Geometry: final body of the model. Coordinates: model frame, mm. Coordinates: 2 decimals unless noted, no trailing zeros. Loops run counter-clockwise (first coordinate to the right, second up) from the corner with the lowest first, then second, coordinate; pieces in that order, holes last. Notation, with made-up numbers: M -13.5,-37.75 L 44.5,-37.75 A19 ccw 44.5,-13.75 Z; hole C 77,2 d6. An arc over 180 degrees is marked long. Write item = value, one per line. Start each with the question number.
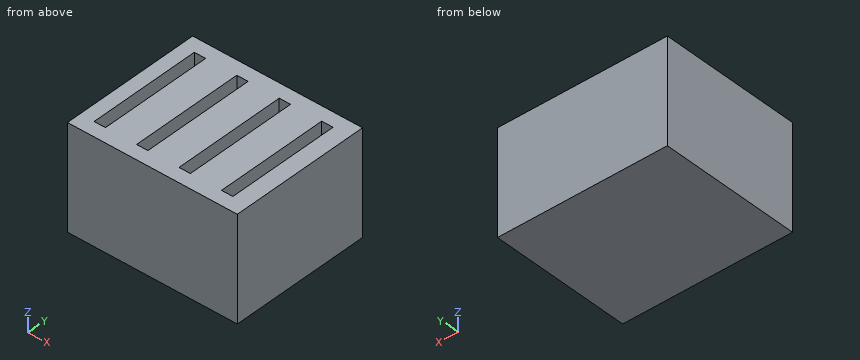
```python
from build123d import *

# Parameters (mm, degrees)
BOX_W        = 2.4
BOX_H        = 24
BOX_DEPTH    = 22
BOX001_W     = 2.4
BOX001_H     = 24
BOX001_DEPTH = 22
BOX002_W     = 2.4
BOX002_H     = 24
BOX002_DEPTH = 22
BOX003_W     = 2.4
BOX003_H     = 24
BOX003_DEPTH = 22
BOX004_W     = 36
BOX004_H     = 30
BOX004_DEPTH = 22


with BuildPart() as box:
    # Box → Box (new body)
    with BuildSketch(Plane.XY):
        with Locations((1.2, 12)):
            Rectangle(BOX_W, BOX_H)
    extrude(amount=BOX_DEPTH)


with BuildPart() as box001:
    # Box001 → Box001 (new body)
    with BuildSketch(Plane(origin=(9, 0, 0), x_dir=(1, 0, 0), z_dir=(0, 0, 1))):
        with Locations((1.2, 12)):
            Rectangle(BOX001_W, BOX001_H)
    extrude(amount=BOX001_DEPTH)


with BuildPart() as box002:
    # Box002 → Box002 (new body)
    with BuildSketch(Plane(origin=(18, 0, 0), x_dir=(1, 0, 0), z_dir=(0, 0, 1))):
        with Locations((1.2, 12)):
            Rectangle(BOX002_W, BOX002_H)
    extrude(amount=BOX002_DEPTH)


with BuildPart() as ranuras:
    # Box003 → Box003 (new body)
    with BuildSketch(Plane(origin=(27, 0, 0), x_dir=(1, 0, 0), z_dir=(0, 0, 1))):
        with Locations((1.2, 12)):
            Rectangle(BOX003_W, BOX003_H)
    extrude(amount=BOX003_DEPTH)

    # Fusion: union Box, Box001, Box002
    add(box.part)
    add(box001.part)
    add(box002.part)


with BuildPart() as ranuras_1:
    # Fusion placement: moved
    add(ranuras.part.moved(Location((0, 0, 3))))


with BuildPart() as cut:
    # Box004 → Box004 (new body)
    with BuildSketch(Plane(origin=(-3, -3, 0), x_dir=(1, 0, 0), z_dir=(0, 0, 1))):
        with Locations((18, 15)):
            Rectangle(BOX004_W, BOX004_H)
    extrude(amount=BOX004_DEPTH)

    # Cut: cut Ranuras
    add(ranuras_1.part, mode=Mode.SUBTRACT)


solid = cut.part
```
Item 1: First-contact query: pin 1 (1.9 mm diameter, centred on x = 28.5, y = 13, fed in from +Z); pin 2 (0.7 mm diameter, centred on x = 10, y = 13, fed in from +Z). Flat tips, straight axial feed; report the tip coordinate or a pass-through.
Item 2: Section query A-A (z = 13.25). Return the cut outline in (x, y), plus the area to 3 significant figures.
Item 3: Line query: line 1 (X direction, y = 8, z = 16.75); line 2 (Y direction, x = 10, z = 15.75). Output: solid intervals per line, ascending. Write a range as from..to.
Item 4: Section query B-B (y = 12.75). Return the cut outline in (x, z).
Item 5: Section query C-C (x = 28.5). Return the cut outline in (y, z), plus the area to 3 significant figures.
Verdict:
q1.pin_1 = 22
q1.pin_2 = 3
q2.outline = M -3,-3 L 33,-3 L 33,27 L -3,27 Z; hole M 0,0 L 2.4,0 L 2.4,24 L 0,24 Z; hole M 9,0 L 11.4,0 L 11.4,24 L 9,24 Z; hole M 18,0 L 20.4,0 L 20.4,24 L 18,24 Z; hole M 27,0 L 29.4,0 L 29.4,24 L 27,24 Z
q2.area = 850 mm2
q3.line_1 = -3..0, 2.4..9, 11.4..18, 20.4..27, 29.4..33
q3.line_2 = -3..0, 24..27
q4.outline = M -3,0 L 33,0 L 33,22 L 29.4,22 L 29.4,3 L 27,3 L 27,22 L 20.4,22 L 20.4,3 L 18,3 L 18,22 L 11.4,22 L 11.4,3 L 9,3 L 9,22 L 2.4,22 L 2.4,3 L 0,3 L 0,22 L -3,22 Z
q5.outline = M -3,0 L 27,0 L 27,22 L 24,22 L 24,3 L 0,3 L 0,22 L -3,22 Z
q5.area = 204 mm2
